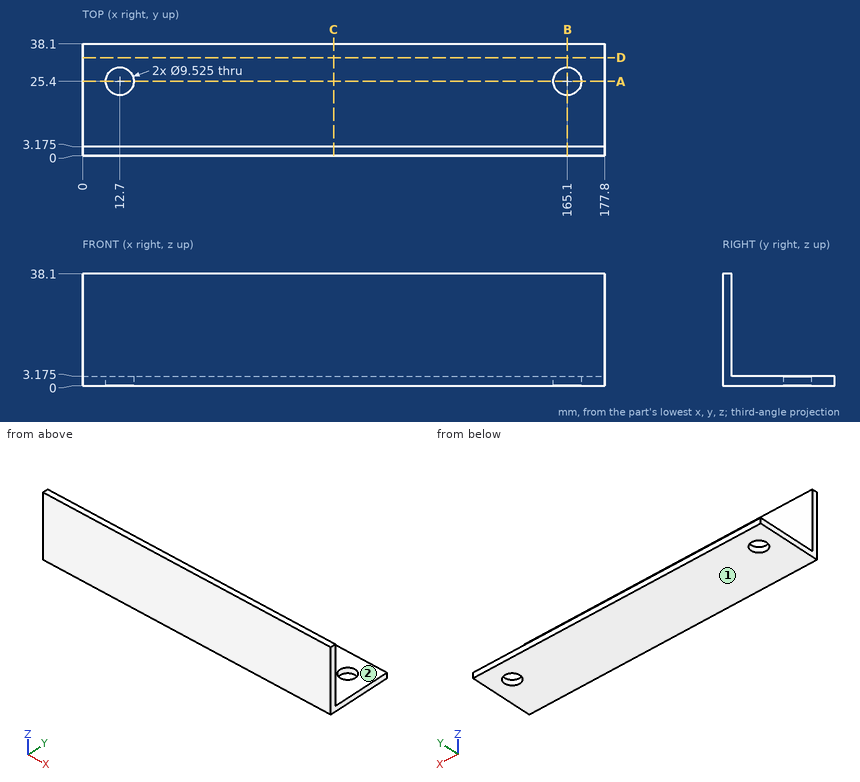
Study the drawing (mm; zero at the part's minimum x, y, z) and answer. A direction names the side the tool comes from. Round coordinates to 2 decimals unless told otherwise and drop trailing zeros. Write each loop counter-clockwise with the first axis right and the second up, starting at its lowest first coordinate (ties: lowest second). Pieces come first, ordered by that corner, then holes.
1) A cutting plane is placed at D-D (y = 33.5). Give the vertices of the cut face in (x, z) (3 decimals), plus the area to 3 significant figures.
2) Straight lines are drawn through the part: line 1 (X direction, y = 25, z = 1); line 2 (Y direction, x = 12.7, z = 1.35); line 3 (Z direction, x = 64.5, y = 35) (3 decimals). For each, find the intervals that lie inside material, in ascending order.
3) Given pin 1 Ø3 at (x, z) = (42.5, 24) entering from +Y (3 decimals); pin 2 Ø10 at (x, y) = (45.5, 25) entering from -Z; pin 3 Ø1 at (x, y) = (42.5, 16) entering from +Z (3 decimals); pin 4 Ø12 at (y, z) = (20, 14) entering from +X, each flat-ended and moving along its own axis, determine where each tip first touches the part or whether it passes through.
4) A tool of negligible diameter and unlimited length cuts with its end or side. For the marked faces 1 and 2, from which of +Z, -Z, +X, -X, +Y, -Y can it reach the whole face along a straight path? Write none if from no direction.
5) A cutting plane is placed at A-A (y = 25.4). Give the vertices of the cut face in (x, z) (1 decimal).
6) A cutting plane is placed at C-C (x = 85.5). Give the vertices of the cut face in (y, z) (3 decimals).
7) A cutting plane is placed at B-B (x = 165.1). Give the vertices of the cut face in (y, z) (1 decimal).
Completed:
1. outline: (0, 0) - (177.8, 0) - (177.8, 3.175) - (0, 3.175) - close
1. area: 565 mm2
2. line 1: x = 0 to 7.95, 17.45 to 160.35, 169.85 to 177.8
2. line 2: y = 0 to 20.64, 30.16 to 38.1
2. line 3: z = 0 to 3.175
3. pin 1: stops at y = 3.175
3. pin 2: stops at z = 0
3. pin 3: stops at z = 3.175
3. pin 4: passes through
4. face 1: -Z, +X, -X, +Y, -Y
4. face 2: +Z, +X, -X, +Y
5. outline: (0, 0) - (7.9, 0) - (7.9, 3.2) - (0, 3.2) - close; (17.5, 0) - (160.3, 0) - (160.3, 3.2) - (17.5, 3.2) - close; (169.9, 0) - (177.8, 0) - (177.8, 3.2) - (169.9, 3.2) - close
6. outline: (0, 0) - (38.1, 0) - (38.1, 3.175) - (3.175, 3.175) - (3.175, 38.1) - (0, 38.1) - close
7. outline: (0, 0) - (20.6, 0) - (20.6, 3.2) - (3.2, 3.2) - (3.2, 38.1) - (0, 38.1) - close; (30.2, 0) - (38.1, 0) - (38.1, 3.2) - (30.2, 3.2) - close
